Geometry check sheet. Reference: the model listing, model coordinates, mm. Face numbers are marked on the shaded views. Coordinates: 2 decimals unless noted, no trailing zeros. Loops run counter-clockwise (first coordinate to the right, second up) from the corner with the lowest first, then second, coordinate; pieces in that order, holes last. Notation, with made-up numbers: (42, 17) -> (66, 17) arc R19 ccw to (66, 21) -> close; hole circle Ø10 at (4, 7.5). An arc over 180 degrees is marked (long way). Answer as a JSON object with one key per item and string values.
from build123d import *

# Parameters (mm, degrees)
F0_R     = 16
F1_DEPTH = 50
F2_R     = 14.5
F3_DEPTH = 35
F4_R     = 8.5
F5_DEPTH = 30
F6_R     = 6.5
F7_DEPTH = 45.001
F8_R     = 10
F9_DEPTH = 8


with BuildPart() as f1:
    # F0 (on Top) → F1 (new body)
    with BuildSketch(Plane.XY):
        Circle(F0_R)
    extrude(amount=F1_DEPTH)

    # F2 (on face) → F3 (cut)
    with BuildSketch(Plane.XY.offset(50)):
        Circle(F2_R)
    extrude(amount=-F3_DEPTH, mode=Mode.SUBTRACT)

    # F4 (on face) → F5 (join)
    with BuildSketch(Plane(origin=(0, 0, 0), x_dir=(1, 0, 0), z_dir=(0, 0, -1))):
        Circle(F4_R)
    extrude(amount=F5_DEPTH)

    # F6 (on face) → F7 (cut, through all)
    with BuildSketch(Plane.XY.offset(15)):
        Circle(F6_R)
    extrude(amount=-F7_DEPTH, mode=Mode.SUBTRACT)

    # F8 (on face) → F9 (cut)
    with BuildSketch(Plane.XY.offset(15)):
        Circle(F8_R)
    extrude(amount=-F9_DEPTH, mode=Mode.SUBTRACT)


solid = f1.part
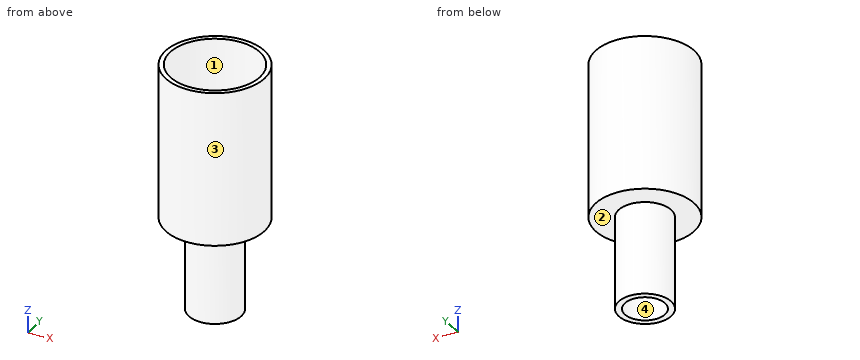
1. Section check C-C, the plane z = -1. Record the boundary of the cut face in (x, y).
Evaluation:
{"outline": "circle Ø17 at (0, 0); hole circle Ø13 at (0, 0)"}
2. Thickness scan on probe 1 along Y at (x, z) = (-0.5, 9.5); probe 2 along Y at (x, z) = (0, -10); probe 3 along X at (y, z) = (-6, -21). Record the ranges inside material, lowest first. Write a range as from..to.
Evaluation:
{"probe 1": "y = -15.99..-9.99, 9.99..15.99", "probe 2": "y = -8.5..-6.5, 6.5..8.5", "probe 3": "x = -6.02..-2.5, 2.5..6.02"}
3. Mould release check, pull along X, two halves, no side actions. Record for the marked faces 1, 2, 3 and 4: released by +X, released by -X, zero draft, split by the parting line, or undercut.
Evaluation:
{"face 1": "undercut", "face 2": "zero draft", "face 3": "split by the parting line", "face 4": "undercut"}
4. Depth check by flat-ended pin: P1, Ø2, axis at y = -11, z = 25.5, coming from the +X side; P2, Ø10, axis at x = 3.5, z = -6.5, coming from the +Y side; P3, Ø1, axis at x = 7, z = -9, coming from the -Y side. Enter the tip coordinate at first touch or a pass-through.
Evaluation:
{"P1": "stops at x = 12.49", "P2": "stops at y = 8.5", "P3": "stops at y = -5.48"}
5. Section check D-D, the plane y = 13. Record the boundary of the cut face in (x, z).
Evaluation:
{"outline": "(-9.33, 0) -> (9.33, 0) -> (9.33, 50) -> (6.42, 50) -> (6.42, 15) -> (-6.42, 15) -> (-6.42, 50) -> (-9.33, 50) -> close"}
6. Section check A-A, the plane x = 0. Record the boundary of the cut face in (y, z), then the cut area to 3 significant figures.
Evaluation:
{"outline": "(-16, 0) -> (-8.5, 0) -> (-8.5, -30) -> (-6.5, -30) -> (-6.5, 7) -> (-10, 7) -> (-10, 15) -> (-14.5, 15) -> (-14.5, 50) -> (-16, 50) -> close; (6.5, -30) -> (8.5, -30) -> (8.5, 0) -> (16, 0) -> (16, 50) -> (14.5, 50) -> (14.5, 15) -> (10, 15) -> (10, 7) -> (6.5, 7) -> close", "area": "454 mm^2"}
